Part model, mm, in its own coordinate system. A direction names the side the tool comes from. Give positions to 0.01 mm unless a question says otherwise; leave off trailing zeros. Write each loop counter-clockwise with the first axis right and the second up, starting at its lowest first coordinate (ties: lowest second). Pieces come first, ordered by that corner, then holes. Notation, with made-up numbers: M 78,60 L 124,60 A20 ccw 124,85 Z; hole C 77,-25 d9. An arc over 180 degrees is marked long. Write item = value, one per line. Start each with the question number.
Autodesk Inventor part; units mm, degrees
ref_plane "YZ Plane" through (0, 0, 0) normal (1, 0, 0) x (0, 1, 0)
ref_plane "XZ Plane" through (0, 0, 0) normal (0, 1, 0) x (-1, 0, 0)
ref_plane "XY Plane" through (0, 0, 0) normal (0, 0, 1) x (1, 0, 0)
sketch "Skizze1" plane through (0, 0, 0) normal (0, 0, 1) x (1, 0, 0)
  circle A0 centre (0, 0) radius 1.5
  circle A1 centre (-20.5, 0) radius 1.8
  circle A2 centre (-20.5, 0) radius 3.9
  line L0 (0, 0) -> (-20.5, 0) construction
  line L1 (0, 6.5) -> (-20.5, 6.5)
  line L2 (-20.5, -6.5) -> (0, -6.5)
  arc A3 (0, -6.5) -> (0, 6.5) centre (0, 0) ccw
  arc A4 (-20.5, 6.5) -> (-20.5, -6.5) centre (-20.5, 0) ccw
  point P0 (-10.25, 0)
  dimension "d0" = 3
  dimension "d1" = 7.8
  dimension "d2" = 13
extrude "Extrusion1" add sketch "Skizze1" along normal blind 8 contours A3 L2 A4 L1
sketch "Skizze2" plane through (0, 0, 0) normal (0, 0, -1) x (-1, 0, 0)
  circle A0 centre (0, 0) radius 1.5
  circle A1 centre (0, 0) radius 3.5
  dimension "d5" = 7
extrude "Extrusion2" cut sketch "Skizze2" against normal blind 6 contours A0 | A1
sketch "Skizze3" plane through (-20.5, 6.5, 0) normal (0, 1, 0) x (1, 0, 0)
  line L0 (3.9, -8) -> (3.9, 0)
  circle A0 centre (5.1112, -4) radius 1.4
  point P0 (20.5, 0)
  dimension "d8" = 2.8
extrude "Extrusion3" cut sketch "Skizze3" against normal through all
properties part number "Holisheet_NEMA8_Syringe_pusher"
Q1. Two-plate mould, pull along Z, no slides. Class faces 1 (the face through (6.5, 0.1, 3.9)), 2 (the face through (-14.096, 0.091, 4.536)), 3 (the face through (0, -2, 6)), 4 (the face through (-10, 0, 8)): +Z half, -Z half, draft (parallel to the pull), parting line (faces both ways), or undercut.
Q2. Slice it at D-D (z = 6.75). Give the cut face in (x, y).
Q3. Slice it at B-B (y = 2). Give the cut face in (x, z), and give its area (3 significant figures).
Q4. Tool access for faces 5 (the face through (-3.233, -1.341, 2.958)), 6 (the face through (-10, -6.5, 4)): list every direction of +Z, -Z, +X, -X, +Y, -Y with a clear straight run to the whole face (end or side of a thin tool).
Q5. Slice it at A-A (z = 5). Give the cut face in (x, y), and give its area (3 significant figures).
Q6. Probe line 1 along X through (y, z) = (-2, 4.5); line 2 along X through (y, z) = (-1.5, 2); line 3 along X through (y, z) = (0.5, 3.5). List the from-to ranges inside material, lowest first.
Q7. Slice it at C-C (x = -17.5). Give the cut face in (y, z), and give its area (3 significant figures).
Q8. Drop a flat-ended pin along its axis: P1, Ø6.5, axis at x = 0, y = 0, coming from the -Z side. Give the stop position or say it passes through.
Working result:
q1.face_1 = draft
q1.face_2 = undercut
q1.face_3 = -Z half
q1.face_4 = +Z half
q2.outline = M -20.5,-6.5 L 0,-6.5 A6.5 ccw 0,6.5 L -20.5,6.5 A6.5 ccw Z; hole C -20.5,0 d7.8; hole C 0,0 d3
q3.outline = M -26.68,0 L -23.85,0 L -23.85,8 L -26.68,8 Z; M -17.15,0 L -2.87,0 L -2.87,6 L 2.87,6 L 2.87,0 L 6.18,0 L 6.18,8 L -17.15,8 Z; hole C -15.39,4 d2.8
q3.area = 169 mm2
q4.face_5 = -Z
q4.face_6 = +Z, -Z, +X, -X, -Y
q5.outline = M -20.5,-6.5 L -16.37,-6.5 L -16.37,6.5 L -20.5,6.5 A6.5 ccw Z; M -14.41,-6.5 L 0,-6.5 A6.5 ccw 0,6.5 L -14.41,6.5 Z; hole C -20.5,0 d7.8; hole C 0,0 d7
q5.area = 287 mm2
q6.line_1 = -26.68 to -23.85, -17.15 to -16.7, -14.08 to -2.87, 2.87 to 6.18
q6.line_2 = -26.82 to -24.1, -16.9 to -3.16, 3.16 to 6.32
q6.line_3 = -26.98 to -24.37, -14.08 to -3.46, 3.46 to 6.48
q7.outline = M -6.5,0 L -2.49,0 L -2.49,8 L -6.5,8 Z; M 2.49,0 L 6.5,0 L 6.5,8 L 2.49,8 Z
q7.area = 64.1 mm2
q8.P1 = 6
